The listing builds one solid part. Answer for the finished solid, in the listing's coordinates (mm). A direction names the side the tool comes from. Coordinates: 2 decimals unless noted, no trailing zeros. Order: outer loops, then holes, each group sorted by start corner. A loop starts at its lowest first (then second) coordinate and runs counter-clockwise, first axis right, second up. Notation, with made-up numbers: (-6.75, 6) -> (25.25, 6) arc R13 ccw to (25.25, 13) -> close; hole circle Ø11 at (24, 14.25). An arc over 180 degrees is marked (long way). Write each question's results on one line, items separated by ' | '. Start each with the question number.
(1) The part is cut by section A-A, the plane y = 10.75. Count the separate pieces of the cut face and the enclosed holes in it, then the cut area to 3 significant figures.
(2) Given pin 1 (4 mm diameter, centred on x = -15, y = 6.5, fed in from -Z); pin 2 (2.5 mm diameter, centred on y = 9.5, z = 20, fed in from -X); pin 3 (5.5 mm diameter, centred on y = 7.5, z = 19.5, fed in from +X), each flat-ended and moving along its own axis, determine where each tip first touches the part or whether it passes through.
(3) A tool of negligible diameter and unlimited length cuts with its end or side. For faces 4 (the face through (-8.356, 7, 19)), 5 (the face through (-14, 7, 30.292)), 6 (the face through (-14, 7, 26.101)), 7 (the face through (1.296, 7, 28)), from which of +Z, -Z, +X, -X, +Y, -Y can it reach the whole face along a straight path? Write none if from no direction.
(4) The part is cut by section B-B, the plane x = -16.5. Give the vertices of the cut face in (y, z).
(5) The part is cut by section C-C, the plane z = 18.25. Give the vertices of the cut face in (x, y), then the cut area to 3 significant figures.
(6) Determine the mould class of faces 1 (the face through (-4, 7, 21.91)), 2 (the face through (-4, 7, 30.292)), 3 (the face through (-3.6, 12.954, 21.1)) for opening direction Z: +Z half, -Z half, draft (parallel to the pull), parting line (faces both ways), or undercut.
(7) The part is cut by section D-D, the plane x = 1. Give the vertices of the cut face in (y, z).
(8) Straight lines are drawn through the part: L1, parallel to Z at x = -13, y = 10.5; L2, parallel to X at y = 1.75, z = 28.75; L3, parallel to Z at x = -8, y = 6.25. For each, find the intervals that lie inside material, in ascending order.
```python
from build123d import *

# Parameters (mm, degrees)
F0_W      = 25.4
F0_H      = 22.86
F1_DEPTH  = 1.016
F2_W      = 6.35
F2_H      = 0.889
F3_DEPTH  = 25.4
F4_W      = 9.652
F4_H      = 5.207
F4_W_2    = 7.62
F4_H_2    = 3.175
F5_DEPTH  = 12.954
F6_W      = 25.4
F6_H      = 2.794
F6_H_2    = 3.048
F7_DEPTH  = 12.955
F8_W      = 2.54
F8_H      = 17.018
F9_DEPTH  = 25.4
F10_DEPTH = 0.508


with BuildPart() as f1:
    # F0 (on Front) → F1 (new body)
    with BuildSketch(Plane.XZ):
        with Locations((-10.1341714823, 23.5612259712)):
            Rectangle(F0_W, F0_H)
    extrude(amount=-F1_DEPTH)

    # F2 (on face) → F3 (cut)
    with BuildSketch(Plane.XZ):
        with Locations((-14.1981714823, 27.6887259712)):
            Rectangle(F2_W, F2_H)
        with Locations((-3.5301714823, 27.6887259712)):
            Rectangle(F2_W, F2_H)
        with Locations((-14.1981714823, 19.1797259712)):
            Rectangle(F2_W, F2_H)
        with Locations((-3.5301714823, 19.1797259712)):
            Rectangle(F2_W, F2_H)
    extrude(amount=-F3_DEPTH, mode=Mode.SUBTRACT)

    # F4 (on face) → F5 (join)
    with BuildSketch(Plane.XZ):
        with Locations((-14.1981714823, 27.6887259712)):
            Rectangle(F4_W, F4_H)
        with Locations((-14.1981714823, 27.6887259712)):
            Rectangle(F4_W_2, F4_H_2, mode=Mode.SUBTRACT)
        with Locations((-3.5301714823, 27.6887259712)):
            Rectangle(F4_W, F4_H)
        with Locations((-3.5301714823, 27.6887259712)):
            Rectangle(F4_W_2, F4_H_2, mode=Mode.SUBTRACT)
        with Locations((-14.1981714823, 19.3067259712)):
            Rectangle(F4_W, F4_H)
        with Locations((-14.1981714823, 19.3067259712)):
            Rectangle(F4_W_2, F4_H_2, mode=Mode.SUBTRACT)
        with Locations((-3.5301714823, 19.3067259712)):
            Rectangle(F4_W, F4_H)
        with Locations((-3.5301714823, 19.3067259712)):
            Rectangle(F4_W_2, F4_H_2, mode=Mode.SUBTRACT)
    extrude(amount=-F5_DEPTH)

    # F6 (on face) → F7 (cut, through all)
    with BuildSketch(Plane.XZ):
        with Locations((-10.1341714823, 13.5282259712)):
            Rectangle(F6_W, F6_H)
        with Locations((-10.1341714823, 33.4672259712)):
            Rectangle(F6_W, F6_H_2)
    extrude(amount=-F7_DEPTH, mode=Mode.SUBTRACT)

    # F8 (on face) → F9 (cut)
    with BuildSketch(Plane.XZ):
        with Locations((-21.5641714823, 23.4342259712)):
            Rectangle(F8_W, F8_H)
    extrude(amount=-F9_DEPTH, mode=Mode.SUBTRACT)

    # F10 (cut): faces of the model
    f10_faces = [f1.faces().sort_by_distance(p)[0] for p in [
        (-14.1981714823, 1.016, 26.1837759712),
        (-3.5301714823, 1.016, 20.8116759712),
        (-14.1981714823, 1.016, 17.8017759712),
        (-7.2576214823, 1.016, 27.6887259712),
    ]]
    extrude(f10_faces, amount=-F10_DEPTH, mode=Mode.SUBTRACT)


solid = f1.part
```
Established:
1) separate pieces: 4 | enclosed holes: 4 | area: 104 mm^2
2) pin 1: stops at z = 16.7 | pin 2: stops at x = -19.02 | pin 3: stops at x = 1.3
3) face 4: +Z, -Z, +Y | face 5: +Z, +X, -X, +Y | face 6: +Y | face 7: +Z, -Z, +X, +Y
4) outline: (0, 14.93) -> (1.02, 14.93) -> (1.02, 16.7) -> (12.95, 16.7) -> (12.95, 17.72) -> (0.51, 17.72) -> (0.51, 18.74) -> (0, 18.74) -> close; (0, 19.62) -> (0.51, 19.62) -> (0.51, 20.89) -> (12.95, 20.89) -> (12.95, 21.91) -> (1.02, 21.91) -> (1.02, 25.09) -> (12.95, 25.09) -> (12.95, 26.1) -> (0.51, 26.1) -> (0.51, 27.24) -> (0, 27.24) -> close; (0, 28.13) -> (0.51, 28.13) -> (0.51, 29.28) -> (12.95, 29.28) -> (12.95, 30.29) -> (1.02, 30.29) -> (1.02, 31.94) -> (0, 31.94) -> close
5) outline: (-20.29, 0) -> (2.57, 0) -> (2.57, 1.02) -> (1.3, 1.02) -> (1.3, 12.95) -> (0.28, 12.95) -> (0.28, 0.51) -> (-7.34, 0.51) -> (-7.34, 12.95) -> (-8.36, 12.95) -> (-8.36, 1.02) -> (-9.37, 1.02) -> (-9.37, 12.95) -> (-10.39, 12.95) -> (-10.39, 0.51) -> (-18.01, 0.51) -> (-18.01, 12.95) -> (-19.02, 12.95) -> (-19.02, 1.02) -> (-20.29, 1.02) -> close | area: 64.0 mm^2
6) face 1: undercut | face 2: +Z half | face 3: draft
7) outline: (0, 14.93) -> (1.02, 14.93) -> (1.02, 16.7) -> (12.95, 16.7) -> (12.95, 21.91) -> (1.02, 21.91) -> (1.02, 25.09) -> (12.95, 25.09) -> (12.95, 30.29) -> (1.02, 30.29) -> (1.02, 31.94) -> (0, 31.94) -> close
8) L1: z = 16.7 to 17.72, 20.89 to 21.91, 25.09 to 26.1, 29.28 to 30.29 | L2: x = -19.02 to -18.01, -10.39 to -9.37, -8.36 to -7.34, 0.28 to 1.3 | L3: z = 16.7 to 21.91, 25.09 to 30.29
